Here's the drawing with two shaded views (mm, measured from the low corner). I have some questions. Round coordinates to 2 decimals unless told otherwise and drop trailing zeros. Loops run counter-clockwise (first coordinate to the right, second up) from the corner with the lowest first, then second, coordinate; pieces in that order, holes last. Notation, with made-up numbers: (-9.75, 65.25) - (30.25, 65.25) arc R30 ccw to (30.25, 88.25) - close; hole circle Ø7 at (16, 36). An arc over 180 degrees is marked (long way). Answer as CSV lines item,"result".
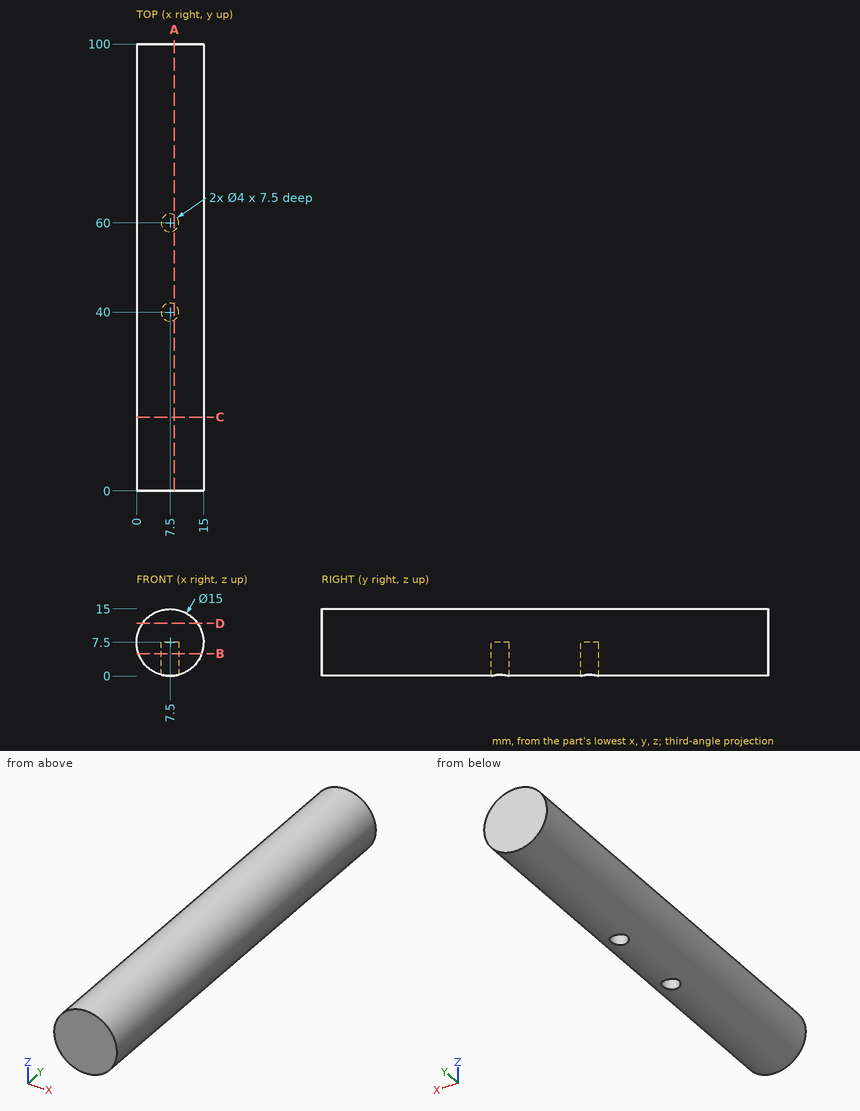
Q1. Imagine slicing it at C-C (y = 16.5). Write out the boundary of the cut face in (x, z), then the cut area to 3 significant figures.
Checks:
outline,"circle Ø15 at (7.5, 7.5)"
area,"177 mm²"
Q2. I'm going to push flat-ended pins straight in: pin 1 Ø5 at (x, y) = (4, 81.5) entering from +Z; pin 2 Ø2 at (x, y) = (7.5, 60.5) entering from -Z; pin 3 Ø2 at (y, z) = (73.5, 1.5) entering from -X. Where does each tip first touch, or does it pass through?
Checks:
pin 1,"z = 14.93"
pin 2,"z = 7.5"
pin 3,"x = 1.91"
Q3. Imagine slicing it at A-A (x = 8.5). Write out the boundary of the cut face in (y, z), then the cut area to 3 significant figures.
Checks:
outline,"(0, 0.07) - (38.27, 0.07) - (38.27, 7.5) - (41.73, 7.5) - (41.73, 0.07) - (58.27, 0.07) - (58.27, 7.5) - (61.73, 7.5) - (61.73, 0.07) - (100, 0.07) - (100, 14.93) - (0, 14.93) - close"
area,"1,440 mm²"
Q4. Imagine slicing it at D-D (z = 11.75). Write out the boundary of the cut face in (x, y), then the cut area to 3 significant figures.
Checks:
outline,"(1.32, 0) - (13.68, 0) - (13.68, 100) - (1.32, 100) - close"
area,"1,240 mm²"
Q5. Imagine slicing it at B-B (z = 5). Write out the boundary of the cut face in (x, y).
Checks:
outline,"(0.43, 0) - (14.57, 0) - (14.57, 100) - (0.43, 100) - close; hole circle Ø4 at (7.5, 40); hole circle Ø4 at (7.5, 60)"
Q6. If I drill on line 1 along Y through (x, z) = (7.5, 4.5); line 2 along Z through (x, y) = (7.75, 70.5); line 3 along X through (y, z) = (32, 14.25), over which ranges is the centre line in solid material (lowest first)? Write a range as [from, to].
Checks:
line 1,"[0, 38], [42, 58], [62, 100]"
line 2,"[0, 15]"
line 3,"[4.23, 10.77]"
